Study the drawing (mm; zero at the part's minimum x, y, z) and answer. A direction names the side the tool comes from. Coordinates: 2 decimals unless noted, no trailing zeros. Loops run counter-clockwise (first coordinate to the right, second up) from the corner with the lowest first, then second, coordinate; pieces in that order, holes last.
Q1. Which of the six approach directions +Z, -Z, +X, -X, +Y, -Y give full straight-line access (tool end or side, diameter ignored) to the marked faces 1, 2, 3, 4 and 5?
Q2. Section C-C (y = 61) is taken. Give the vertices of the cut face in (x, z).
Q3. The mould has two halves that part along X. Classify the marked faces 6, 7 and 8: pulls with the +X half, pulls with the -X half, needs draft (parallel to the pull), parting line crosses it, or undercut.
Q4. Section D-D (x = 44) is taken. Give the vertices of the cut face in (y, z).
Q5. Flat-ended cylindrical pins translate along their axes: P1, Ø2.5, axis at x = 3, z = 3.5, coming from the +Y side; P2, Ø1.5, axis at x = 12.5, z = 2.5, coming from the -Y side; P3, Ø2.5, axis at y = 10, z = 1.5, coming from the +X side. Find the tip coordinate at first contact, or state that the pin passes through.
Q6. Section A-A (y = 16) is taken. Give the vertices of the cut face in (x, z), then the cut area to 3 significant figures.
Q7. Section B-B (z = 3) is taken. Give the vertices of the cut face in (x, y), then the cut area to 3 significant figures.
Q8. Straight lines are drawn through the part: line 1 (X direction, y = 46, z = 1.6); line 2 (X direction, y = 4.5, z = 2.35); line 3 (Y direction, x = 7.5, z = 0.75). For each, find the intervals that lie inside material, in ascending order.
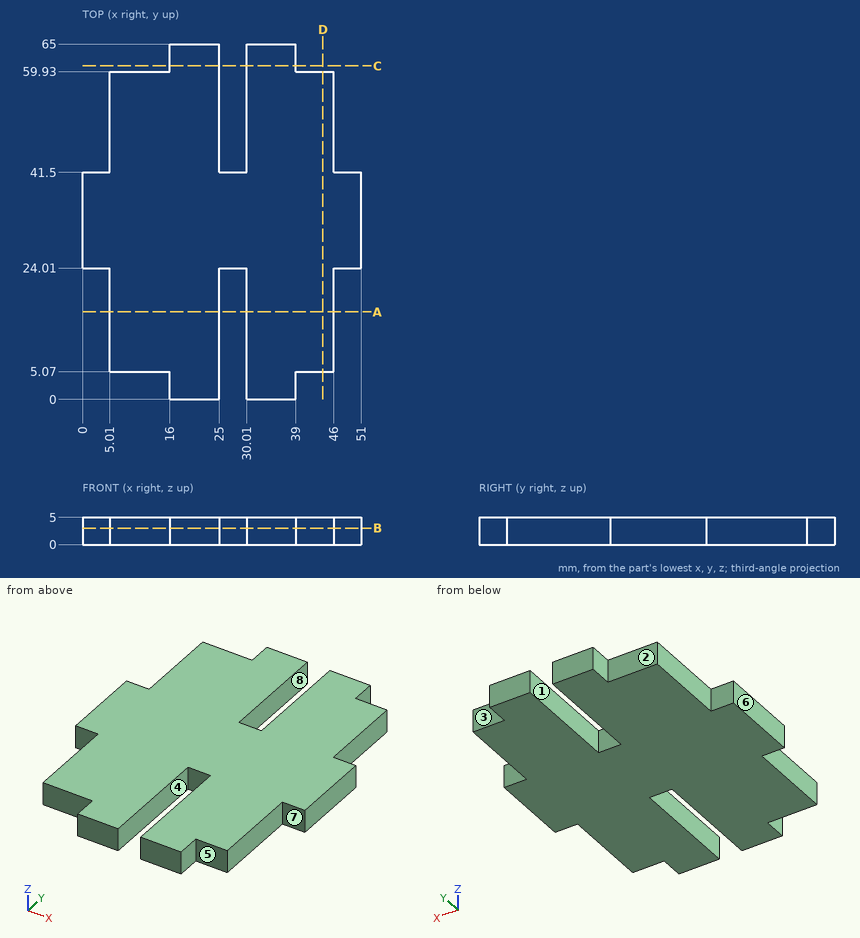
Numbers:
1. face 1: +Z, -Z, +Y
1. face 2: +Z, -Z, -X, +Y
1. face 3: +Z, -Z, +X, +Y
1. face 4: +Z, -Z, -Y
1. face 5: +Z, -Z, +X, -Y
2. outline: (16, 0) - (25, 0) - (25, 5) - (16, 5) - close; (30.01, 0) - (39, 0) - (39, 5) - (30.01, 5) - close
3. face 6: pulls with the -X half
3. face 7: needs draft
3. face 8: undercut
4. outline: (5.07, 0) - (59.93, 0) - (59.93, 5) - (5.07, 5) - close
5. P1: stops at y = 41.5
5. P2: stops at y = 5.07
5. P3: stops at x = 46
6. outline: (5.01, 0) - (25, 0) - (25, 5) - (5.01, 5) - close; (30.01, 0) - (46, 0) - (46, 5) - (30.01, 5) - close
6. area: 180 mm2
7. outline: (0, 24.01) - (5.01, 24.01) - (5.01, 5.07) - (16, 5.07) - (16, 0) - (25, 0) - (25, 24.01) - (30.01, 24.01) - (30.01, 0) - (39, 0) - (39, 5.07) - (46, 5.07) - (46, 24.01) - (51, 24.01) - (51, 41.5) - (46, 41.5) - (46, 59.93) - (39, 59.93) - (39, 65) - (30.01, 65) - (30.01, 41.5) - (25, 41.5) - (25, 65) - (16, 65) - (16, 59.93) - (5.01, 59.93) - (5.01, 41.5) - (0, 41.5) - close
7. area: 2,420 mm2
8. line 1: x = 5.01 to 25, 30.01 to 46
8. line 2: x = 16 to 25, 30.01 to 39
8. line 3: y = 5.07 to 59.93
